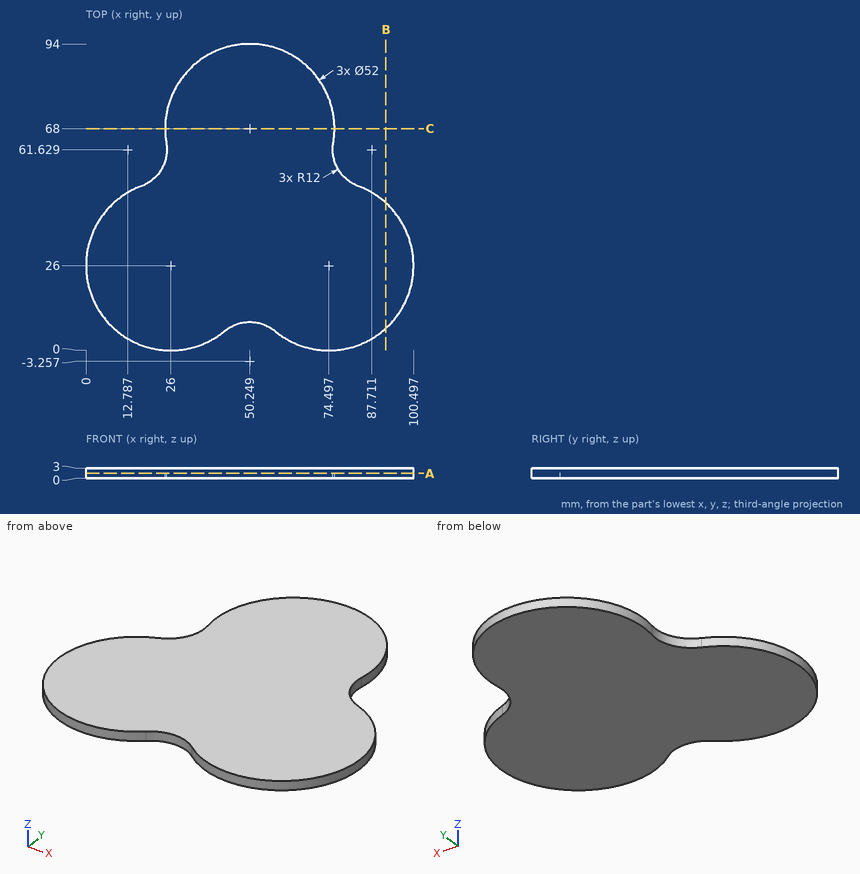
Verification items for this drawing (mm, ordinates from the low corner). Give positions to 0.01 mm unless a question says otherwise; leave off trailing zeros. Write each loop counter-clockwise with the first axis right and the second up, starting at its lowest first coordinate (ties: lowest second). Pieces come first, ordered by that corner, then holes. Notation, with made-up numbers: (62, 45.25) -> (111, 45.25) arc R13 ccw to (111, 52.25) -> close; hole circle Ø11 at (-29.5, 76). An arc over 180 degrees is marked (long way). Use CSV: the item, a comma, the result in double quotes.
(1) Material ranges on L1, parallel to X at y = 68.5, z = 0.45; L2, parallel to X at y = 74, z = 2.05; L3, parallel to Y at x = 21, z = 1.1 (1 decimal), recorded low to high.
Derived:
L1,"x = 24.25 to 76.24"
L2,"x = 24.95 to 75.55"
L3,"y = 0.5 to 52.9"
(2) Sectioned sample at B-B (x = 92). Record the cut outline in (y, z).
Derived:
outline,"(6.77, 0) -> (45.23, 0) -> (45.23, 3) -> (6.77, 3) -> close"
(3) Go/stop test with a flat-tipped pin: pin 1 (1.5 mm diameter, centred on x = 85, z = 2, fed in from -Y). Record where the tip stops, or that it passes through.
Derived:
pin 1,"stops at y = 1.9"
(4) Sectioned sample at A-A (z = 1.5). Record the cut outline in (x, y), plus the area to 4 significant figures.
Derived:
outline,"(16.96, 50.38) arc R26 ccw (long way) to (42.59, 5.98) arc R12 cw to (57.91, 5.98) arc R26 ccw (long way) to (83.54, 50.38) arc R12 cw to (75.88, 63.64) arc R26 ccw (long way) to (24.62, 63.64) arc R12 cw to start"
area,"6,375 mm^2"
(5) Sectioned sample at C-C (y = 68). Record the cut outline in (x, z).
Derived:
outline,"(24.25, 0) -> (76.25, 0) -> (76.25, 3) -> (24.25, 3) -> close"
